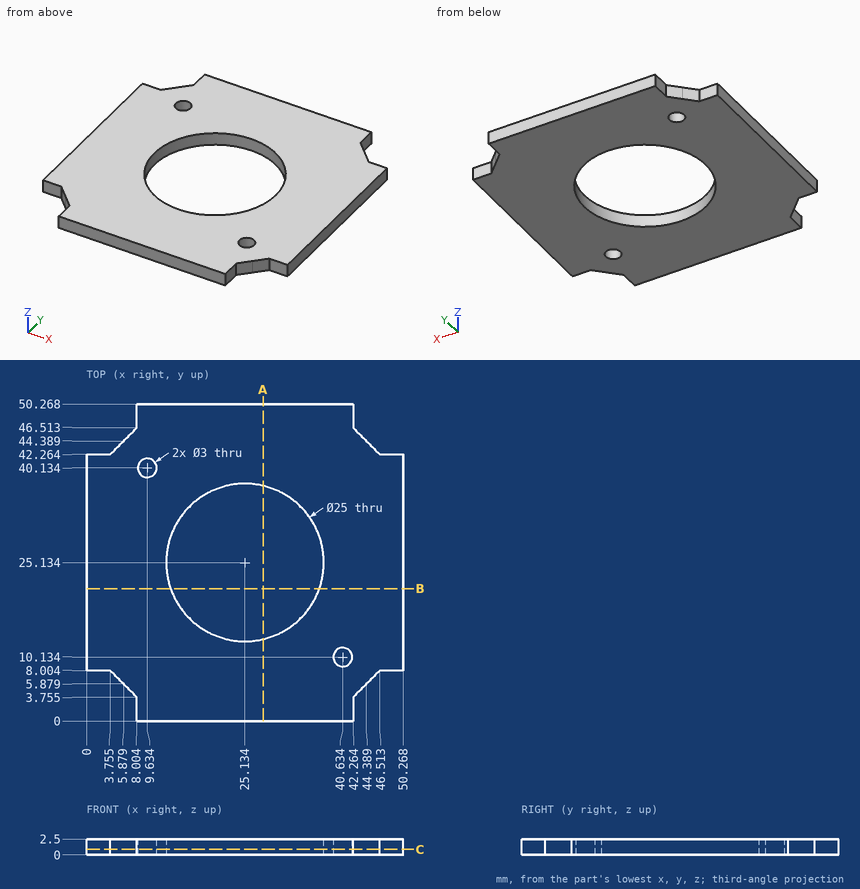
Check sheet for the drawn part. Datum: minimum x, y, z corner. Units: mm. Round coordinates to 2 decimals unless told otherwise and drop trailing zeros. Write each loop counter-clockwise with the first axis right and the second up, starting at its lowest first coordinate (ties: lowest second). Pieces come first, ordered by that corner, then holes. Notation, with made-up numbers: (47.5, 81.5) - (70.5, 81.5) arc R27 ccw to (70.5, 110.5) - close; hole circle Ø1 at (23, 47.5). An arc over 180 degrees is marked (long way). Write each question's results on one line, items separated by ' | '.
(1) Sectioned sample at C-C, the plane z = 0.85. Enter the section's corners in (x, y) (1 decimal).
Computed:
outline: (0, 8) - (3.8, 8) - (5.9, 5.9) - (8, 3.8) - (8, 0) - (42.3, 0) - (42.3, 3.8) - (44.4, 5.9) - (46.5, 8) - (50.3, 8) - (50.3, 42.3) - (46.5, 42.3) - (44.4, 44.4) - (42.3, 46.5) - (42.3, 50.3) - (8, 50.3) - (8, 46.5) - (5.9, 44.4) - (3.8, 42.3) - (0, 42.3) - close; hole circle Ø3 at (9.6, 40.1); hole circle Ø25 at (25.1, 25.1); hole circle Ø3 at (40.6, 10.1)
(2) Sectioned sample at A-A, the plane x = 28. Enter the section's corners in (y, z).
Computed:
outline: (0, 0) - (12.97, 0) - (12.97, 2.5) - (0, 2.5) - close; (37.3, 0) - (50.27, 0) - (50.27, 2.5) - (37.3, 2.5) - close
(3) Sectioned sample at B-B, the plane y = 21. Enter the section's corners in (x, z).
Computed:
outline: (0, 0) - (13.34, 0) - (13.34, 2.5) - (0, 2.5) - close; (36.93, 0) - (50.27, 0) - (50.27, 2.5) - (36.93, 2.5) - close
(4) Depth check by flat-ended pin: pin 1 Ø1.2 at (x, z) = (1, 2) entering from -Y; pin 2 Ø0.8 at (y, z) = (2.5, 1.5) entering from -X. Enter the tip coordinate at first touch or a pass-through.
Computed:
pin 1: stops at y = 8 | pin 2: stops at x = 8
(5) Thickness scan on probe 1 along Y at (x, z) = (40.5, 1.85); probe 2 along X at (y, z) = (24.5, 1.05); probe 3 along X at (y, z) = (2, 0.8). Record the ranges inside material, lowest first. Write a range as from..to.
Computed:
probe 1: y = 0..8.64, 11.63..50.27 | probe 2: x = 0..12.65, 37.62..50.27 | probe 3: x = 8..42.26
